Could you check a few things on this model? Use its own coordinates, in mm. A direction names the side the tool comes from. Round coordinates to 2 decimals unless told otherwise and drop trailing zeros. Loops run counter-clockwise (first coordinate to the right, second up) from the corner with the lowest first, then second, coordinate; pieces in that order, holes last. Notation, with made-up numbers: (69, -20) -> (85, -20) arc R26 cw to (85, 0) -> close; hole circle Ø5 at (63.5, 66.25). An arc over 180 degrees is marked (long way). Put each result on its own line as item: value. Start each with the question number.
1. I need wall thicknesses on line 1 (X direction, y = -25, z = 4.25); line 2 (Z direction, x = -24.5, y = 34); line 3 (Z direction, x = -74.5, y = -48). Which ranges of each line are inside material? Lowest first, please. Write a range as [from, to].
2. If we mould it in two halves opening along X, with no side actions, what happens to faces 1 (the flat face through (-64.95, -54.82, 6.16)), 2 (the flat face through (-1, -1, 0)), 3 (the flat face through (59.75, 34.25, 6.16))? For each: pulls with the +X half, pulls with the -X half, needs draft (parallel to the pull), parting line crosses it, or undercut.
3. Which directions (+Z, -Z, +X, -X, +Y, -Y) give clear straight access to the entire face, cutting with the end or side of a thin tool? Please do faces 4 (the flat face through (64.95, 54.82, 6.16)), 5 (the flat face through (-73, 43, 12.5)), 6 (the flat face through (-1, 1, 15)), 7 (the flat face through (-15, -84, 6)).
4. I'm going to push flat-ended pins straight in: P1, Ø8, axis at y = -61.5, z = 17.5, coming from the +X side; P2, Ø3, axis at y = 9.5, z = 4, coming from the -X side; P3, Ø6, axis at y = 89.5, z = 9, coming from the +X side. Where does each tip first touch, or does it pass through?
5. Imagine slicing it at A-A, the plane z = 4.75. Please give me the cut outline in (x, y).
6. Imagine slicing it at D-D, the plane z = 22.25. Please give me the cut outline in (x, y), and give its area (3 significant figures).
7. Imagine slicing it at B-B, the plane y = 0. Please give me the cut outline in (x, z).
8. Imagine slicing it at C-C, the plane x = 0. Please give me the cut outline in (y, z), and give its area (3 significant figures).
```python
from build123d import *

# Parameters (mm, degrees)
SKETCH1_R           = 100
SKETCH1_R_2         = 60
BOSS_EXTRUDE1_DEPTH = 25
CUT_EXTRUDE1_START  = 25
SKETCH1_3_R         = 60
CUT_EXTRUDE1_DEPTH  = 10
CHAMFER1_SIZE       = 10
CUT_EXTRUDE2_DEPTH  = 12.5
CIRPATTERN1_COUNT   = 6


with BuildPart() as part:
    # Sketch1 → Boss-Extrude1 (new body)
    # profile 1 of 2: a face of its own
    with BuildSketch(Plane(origin=(0, 0, 0), x_dir=(0, 1, 0), z_dir=(0, 0, 1))):
        with Locations(Location((0, 0, 0), (0, 0, 270))):
            Circle(SKETCH1_R)
        Circle(SKETCH1_R_2, mode=Mode.SUBTRACT)
    # profile 2 of 2: a face of its own
    with BuildSketch(Plane(origin=(0, 0, 0), x_dir=(0, 1, 0), z_dir=(0, 0, 1))):
        Circle(SKETCH1_R_2)
    extrude(amount=BOSS_EXTRUDE1_DEPTH)

    # Sketch1<3> → Cut-Extrude1 (cut)
    with BuildSketch(Plane(origin=(0, 0, 0), x_dir=(0, 1, 0), z_dir=(0, 0, 1)).offset(CUT_EXTRUDE1_START)):
        with Locations(Location((0, 0, 0), (0, 0, 270))):
            Circle(SKETCH1_3_R)
    extrude(amount=-CUT_EXTRUDE1_DEPTH, mode=Mode.SUBTRACT)

    # Chamfer1
    chamfer1_edges = [part.edges().sort_by_distance(p)[0] for p in [
        (-100, 0, 25),
    ]]
    chamfer(chamfer1_edges, length=CHAMFER1_SIZE)

    # Sketch3 → Cut-Extrude2 (cut)
    with BuildSketch(Plane(origin=(0, 0, 0), x_dir=(1, 0, 0), z_dir=(0, 0, -1))):
        with BuildLine():
            Line((-15, 98.868599666), (-15, 68.868599666))
            Line((-15, 68.868599666), (15, 68.868599666))
            Line((15, 68.868599666), (15, 98.868599666))
            ThreePointArc((15, 98.868599666), (0, 100), (-15, 98.868599666))
        make_face()
    cut_extrude2 = extrude(amount=-CUT_EXTRUDE2_DEPTH, mode=Mode.SUBTRACT)

    # CirPattern1: Cut-Extrude2 ×6 about axis
    cirpattern1_axis = Axis((0, 0, 0), (0, 0, 1))
    for i in range(1, CIRPATTERN1_COUNT):
        add(cut_extrude2.rotate(cirpattern1_axis, i * 360 / CIRPATTERN1_COUNT), mode=Mode.SUBTRACT)


solid = part.part
```
Entries:
1. line 1: [-96.82, -73.3], [-65.09, 65.09], [73.3, 96.82]
1. line 2: [0, 15]
1. line 3: [12.5, 25]
2. face 1: pulls with the -X half
2. face 2: needs draft
2. face 3: undercut
3. face 4: -Z, +X
3. face 5: -Z
3. face 6: +Z
3. face 7: -Z, -Y
4. P1: x = 81.19
4. P2: x = -99.68
4. P3: x = 50.18
5. outline: (-93.12, -36.44) -> (-67.14, -21.44) -> (-52.14, -47.42) -> (-78.12, -62.42) arc R100 ccw to (-15, -98.87) -> (-15, -68.87) -> (15, -68.87) -> (15, -98.87) arc R100 ccw to (78.12, -62.42) -> (52.14, -47.42) -> (67.14, -21.44) -> (93.12, -36.44) arc R100 ccw to (93.12, 36.44) -> (67.14, 21.44) -> (52.14, 47.42) -> (78.12, 62.42) arc R100 ccw to (15, 98.87) -> (15, 68.87) -> (-15, 68.87) -> (-15, 98.87) arc R100 ccw to (-78.12, 62.42) -> (-52.14, 47.42) -> (-67.14, 21.44) -> (-93.12, 36.44) arc R100 ccw to start
6. outline: circle Ø185.5 at (0, 0); hole circle Ø120 at (0, 0)
6. area: 15,700 mm^2
7. outline: (-100, 0) -> (100, 0) -> (100, 15) -> (90, 25) -> (60, 25) -> (60, 15) -> (-60, 15) -> (-60, 25) -> (-90, 25) -> (-100, 15) -> close
8. outline: (-100, 12.5) -> (-68.87, 12.5) -> (-68.87, 0) -> (68.87, 0) -> (68.87, 12.5) -> (100, 12.5) -> (100, 15) -> (90, 25) -> (60, 25) -> (60, 15) -> (-60, 15) -> (-60, 25) -> (-90, 25) -> (-100, 15) -> close
8. area: 2,920 mm^2
